For this review, take the finished solid that the model builds, in its own axes (mm). A direction names the side the tool comes from. Round coordinates to 2 decimals unless told otherwise and drop trailing zeros. Loops run counter-clockwise (first coordinate to the right, second up) from the corner with the lowest first, then second, coordinate; pieces in that order, holes last. Notation, with made-up numbers: (82.25, -23) -> (103.25, -23) arc R17 cw to (103.25, 6) -> close; hole circle Ø1 at (22.25, 29.5). An arc over 180 degrees is marked (long way). Write each question's results on one line, items separated by ' | '.
```python
from build123d import *

# Parameters (mm, degrees)
SALIENTE_EXTRUIR1_DEPTH = 24
SALIENTE_EXTRUIR2_DEPTH = 8
CROQUIS3_R              = 3.15
SALIENTE_EXTRUIR3_DEPTH = 55.4
CHAFL_N1_SIZE           = 1.2
CHAFL_N1_SIZE2          = 0.692820323


with BuildPart() as part:
    # Croquis1 → Saliente-Extruir1 (new body)
    with BuildSketch(Plane.XY):
        with BuildLine():
            Line((0.57794053, 7.728420585), (63.919718915, 2.991646678))
            ThreePointArc((63.919718915, 2.991646678), (66.696, 0), (63.919718915, -2.991646678))
            Line((63.919718915, -2.991646678), (0.57794053, -7.728420585))
            ThreePointArc((0.57794053, -7.728420585), (-7.75, 0), (0.57794053, 7.728420585))
        make_face()
    extrude(amount=SALIENTE_EXTRUIR1_DEPTH)

    # Croquis2 → Saliente-Extruir2 (add)
    with BuildSketch(Plane.XY):
        with BuildLine():
            Line((0.63014161, -8.426471477), (63.971919995, -3.68969757))
            ThreePointArc((63.971919995, -3.68969757), (67.396, 0), (63.971919995, 3.68969757))
            Line((63.971919995, 3.68969757), (0.63014161, 8.426471477))
            ThreePointArc((0.63014161, 8.426471477), (-8.45, 0), (0.63014161, -8.426471477))
        make_face()
        with BuildLine():
            Line((63.919718915, 2.991646678), (0.57794053, 7.728420585))
            ThreePointArc((0.57794053, 7.728420585), (-7.75, 0), (0.57794053, -7.728420585))
            Line((0.57794053, -7.728420585), (63.919718915, -2.991646678))
            ThreePointArc((63.919718915, -2.991646678), (66.696, 0), (63.919718915, 2.991646678))
        make_face(mode=Mode.SUBTRACT)
    extrude(amount=SALIENTE_EXTRUIR2_DEPTH)

    # Croquis3 → Saliente-Extruir3 (add)
    with BuildSketch(Plane(origin=(0, 0, 0), x_dir=(-1, 0, 0), z_dir=(0, 0, -1))):
        with Locations(Location((0, 0, 0), (0, 0, 180))):
            Circle(CROQUIS3_R)
    extrude(amount=SALIENTE_EXTRUIR3_DEPTH)

    # Chafl_n1
    chafl_n1_edges = [part.edges().sort_by_distance(p)[0] for p in [
        (-3.15, 0, -55.4),
    ]]
    chafl_n1_side = [part.faces().sort_by_distance(p)[0] for p in [
        (-3.15, 0, -27.7),
    ]]
    chamfer(chafl_n1_edges, length=CHAFL_N1_SIZE, length2=CHAFL_N1_SIZE2, reference=chafl_n1_side[0])


solid = part.part
```
1. Consider section C-C (z = -24). State the section outline as (x, y) points, plus the area to 3 significant figures.
Values found:
outline: circle Ø6.3 at (0, 0) | area: 31.2 mm2
2. To check wall thickness, follow probe 1 along Z at (x, y) = (20, 0.25); probe 2 along Y at (x, z) = (-1, -27); probe 3 along Z at (x, y) = (43, -4.75). State the ranges of each line that lie inside material, in increasing order.
Values found:
probe 1: z = 0 to 24 | probe 2: y = -2.99 to 2.99 | probe 3: z = 0 to 8
3. Consider section A-A (y = 0). State the section outline as (x, z) points.
Values found:
outline: (-8.45, 0) -> (-3.15, 0) -> (-3.15, -54.2) -> (-2.46, -55.4) -> (2.46, -55.4) -> (3.15, -54.2) -> (3.15, 0) -> (67.4, 0) -> (67.4, 8) -> (66.7, 8) -> (66.7, 24) -> (-7.75, 24) -> (-7.75, 8) -> (-8.45, 8) -> close
4. Consider section B-B (x = 12). State the section outline as (y, z) points.
Values found:
outline: (-7.58, 0) -> (7.58, 0) -> (7.58, 8) -> (6.87, 8) -> (6.87, 24) -> (-6.87, 24) -> (-6.87, 8) -> (-7.58, 8) -> close
5. Tool access review of faces 1 (the face through (-0.683, 3.075, -26.721)), 2 (the face through (31.805, 5.393, 15.888)), 3 (the face through (32.692, -5.327, 15.888)), 4 (the face through (66.695, 0.063, 15.888)): name each direction out of +Z, -Z, +X, -X, +Y, -Y from which nothing blocks a thin tool from reaching the whole face with its end or side.
Values found:
face 1: -Z | face 2: +Z, +X, +Y | face 3: +Z, +X, -Y | face 4: +Z, +X
6. Consider section D-D (x = 56). State the section outline as (y, z) points, plus the area to 3 significant figures.
Values found:
outline: (-4.29, 0) -> (4.29, 0) -> (4.29, 8) -> (3.58, 8) -> (3.58, 24) -> (-3.58, 24) -> (-3.58, 8) -> (-4.29, 8) -> close | area: 183 mm2
7. For pin 1 (8 mm diameter, centred on y = 0, z = -39, fed in from -X); pin 2 (8 mm diameter, centred on x = 56.5, z = 15.5, fed in from -Y); pin 3 (1 mm diameter, centred on x = 44, y = 3.5, fed in from -Z), all flat-tipped, find the tip position at first contact; note any pin that passes through.
Values found:
pin 1: stops at x = -3.15 | pin 2: stops at y = -3.85 | pin 3: stops at z = 0
